```python
from build123d import *

# Parameters (mm, degrees)
SKETCH1_R                = 3.5
SKETCH1_R_2              = 1.5
SKETCH1_W                = 42
SKETCH1_H                = 22
BOSS_EXTRUDE1_DEPTH      = 10
CUT_EXTRUDE1_START       = 7
SKETCH2_R                = 3
CUT_EXTRUDE1_DEPTH       = 3
BOSS_EXTRUDE2_START      = -15
SKETCH4_R                = 5
BOSS_EXTRUDE2_DEPTH      = 10
BOSS_EXTRUDE3_DEPTH      = 15
BOSS_EXTRUDE3_DEPTH_BACK = 25
SKETCH4_3_R              = 5
SKETCH1_3_R              = 3.5
BOSS_EXTRUDE4_DEPTH      = 4
BOSS_EXTRUDE5_START      = -15
BOSS_EXTRUDE5_DEPTH      = 10
BOSS_EXTRUDE6_DEPTH      = 15
BOSS_EXTRUDE6_DEPTH_BACK = 25
SKETCH6_R                = 5
SKETCH6_R_2              = 3.5
BOSS_EXTRUDE7_START      = -19
SKETCH6_2_R              = 3.5
BOSS_EXTRUDE7_DEPTH      = 28


with BuildPart() as part:
    # Sketch1 → Boss-Extrude1 (new body)
    with BuildSketch(Plane.XY):
        Polygon((34, -15), (-29, -15), (-29, 15), (34, 15), (41.5, 15), (41.5, 7.5), (41.5, -7.5), (41.5, -15), align=None)
        with Locations((34, -7.5)):
            Circle(SKETCH1_R, mode=Mode.SUBTRACT)
        with Locations((34, 7.5)):
            Circle(SKETCH1_R, mode=Mode.SUBTRACT)
        with Locations((24.3, 5)):
            Circle(SKETCH1_R_2, mode=Mode.SUBTRACT)
        with Locations((24.3, -5)):
            Circle(SKETCH1_R_2, mode=Mode.SUBTRACT)
        with Locations(Location((-24.3, -5, 0), (0, 0, 180))):
            Circle(SKETCH1_R_2, mode=Mode.SUBTRACT)
        with Locations(Location((-24.3, 5, 0), (0, 0, 180))):
            Circle(SKETCH1_R_2, mode=Mode.SUBTRACT)
        Rectangle(SKETCH1_W, SKETCH1_H, mode=Mode.SUBTRACT)
    extrude(amount=BOSS_EXTRUDE1_DEPTH)

    # Sketch2 → Cut-Extrude1 (cut)
    with BuildSketch(Plane.XY.offset(CUT_EXTRUDE1_START)):
        with Locations((-24.3, 5)):
            Circle(SKETCH2_R)
        with Locations((-24.3, -5)):
            Circle(SKETCH2_R)
        with Locations((24.3, 5)):
            Circle(SKETCH2_R)
        with Locations((24.3, -5)):
            Circle(SKETCH2_R)
    extrude(amount=CUT_EXTRUDE1_DEPTH, mode=Mode.SUBTRACT)

    # Sketch4 → Boss-Extrude2 (add)
    # profile 1 of 3: a face of its own
    with BuildSketch(Plane(origin=(0, 0, 0), x_dir=(1, 0, 0), z_dir=(0, 1, 0)).offset(BOSS_EXTRUDE2_START)):
        with BuildLine():
            Line((41.5, 0), (41.5, 7))
            ThreePointArc((41.5, 7), (34.5, 14), (27.5, 7))
            Line((27.5, 7), (27.5, 0))
            Line((27.5, 0), (41.5, 0))
        make_face()
        with Locations((34.5, 7)):
            Circle(SKETCH4_R, mode=Mode.SUBTRACT)
    # profile 2 of 3: a face of its own
    with BuildSketch(Plane(origin=(0, 0, 0), x_dir=(1, 0, 0), z_dir=(0, 1, 0)).offset(BOSS_EXTRUDE2_START)):
        Polygon((-29, -10), (-29, 0), (27.5, 0), (41.5, 0), (41.5, -10), align=None)
    # profile 3 of 3: a face of its own
    with BuildSketch(Plane(origin=(0, 0, 0), x_dir=(1, 0, 0), z_dir=(0, 1, 0)).offset(BOSS_EXTRUDE2_START)):
        with BuildLine():
            Line((-29, 0), (-9.952221542, 0))
            ThreePointArc((-9.952221542, 0), (-7.49675311, 23.163932944), (6.211711403, 41.99675311))
            Line((6.211711403, 41.99675311), (3.068568225, 45.885281233))
            ThreePointArc((3.068568225, 45.885281233), (-16.210887038, 25.210644422), (-29, 0))
        make_face()
    extrude(amount=-BOSS_EXTRUDE2_DEPTH)

    # Sketch4<3> → Boss-Extrude3 (add, two sides: drawn at the far end of the back side and taken through both)
    with BuildSketch(Plane(origin=(0, 0, 0), x_dir=(1, 0, 0), z_dir=(0, 1, 0)).offset(-BOSS_EXTRUDE3_DEPTH_BACK)):
        with BuildLine():
            Line((41.5, 0), (41.5, 7))
            ThreePointArc((41.5, 7), (34.5, 14), (27.5, 7))
            Line((27.5, 7), (27.5, 0))
            Line((27.5, 0), (41.5, 0))
        make_face()
        with Locations((34.5, 7)):
            Circle(SKETCH4_3_R, mode=Mode.SUBTRACT)
    extrude(amount=BOSS_EXTRUDE3_DEPTH + BOSS_EXTRUDE3_DEPTH_BACK)

    # Sketch1<3> → Boss-Extrude4 (add)
    with BuildSketch(Plane.XY):
        with Locations((34, 7.5)):
            Circle(SKETCH1_3_R)
        with Locations((34, -7.5)):
            Circle(SKETCH1_3_R)
    extrude(amount=BOSS_EXTRUDE4_DEPTH)

    # Sketch5 → Boss-Extrude5 (add)
    with BuildSketch(Plane(origin=(0, 0, 0), x_dir=(1, 0, 0), z_dir=(0, 1, 0)).offset(BOSS_EXTRUDE5_START)):
        with BuildLine():
            Line((-7.556310354, 0), (-29, 0))
            ThreePointArc((-29, 0), (-16.210887038, 25.210644422), (3.068568225, 45.885281233))
            ThreePointArc((3.068568225, 45.885281233), (14.95066501, 52.529162568), (28.36797257, 54.831604973))
            Line((28.36797257, 54.831604973), (28.36797257, 51.580244948))
            Line((28.36797257, 51.580244948), (28.36797257, 49.056310354))
            ThreePointArc((28.36797257, 49.056310354), (27.851378801, 48.977742164), (27.335790025, 48.892828699))
            ThreePointArc((27.335790025, 48.892828699), (26.606861218, 46.521101207), (26.177213589, 44.077368115))
            ThreePointArc((26.177213589, 44.077368115), (25.629076173, 43.950056975), (25.082884112, 43.814642852))
            ThreePointArc((25.082884112, 43.814642852), (23.590633664, 45.796969038), (21.864411592, 47.579266955))
            ThreePointArc((21.864411592, 47.579266955), (21.366468722, 47.420852999), (20.870511092, 47.256329106))
            ThreePointArc((20.870511092, 47.256329106), (20.521576529, 44.799771926), (20.479502655, 42.318913548))
            ThreePointArc((20.479502655, 42.318913548), (19.95802957, 42.107422235), (19.439745475, 41.888232022))
            ThreePointArc((19.439745475, 41.888232022), (17.65576297, 43.612713083), (15.671980735, 45.103027328))
            ThreePointArc((15.671980735, 45.103027328), (15.204949771, 44.868668285), (14.740835409, 44.628585087))
            ThreePointArc((14.740835409, 44.628585087), (14.780487018, 42.147686811), (15.127022896, 39.690790112))
            ThreePointArc((15.127022896, 39.690790112), (14.645054541, 39.400326245), (14.167440286, 39.102757132))
            ThreePointArc((14.167440286, 39.102757132), (12.135653294, 40.526930621), (9.943158199, 41.688564712))
            ThreePointArc((9.943158199, 41.688564712), (9.518538992, 41.384031278), (9.097695935, 41.074300421))
            ThreePointArc((9.097695935, 41.074300421), (9.524957362, 38.630148998), (10.251570129, 36.257710929))
            ThreePointArc((10.251570129, 36.257710929), (9.820974163, 35.895426693), (9.395790198, 35.526805819))
            ThreePointArc((9.395790198, 35.526805819), (7.166228058, 36.615603857), (4.819006607, 37.419954507))
            ThreePointArc((4.819006607, 37.419954507), (4.447254693, 37.052745307), (4.080045493, 36.680993393))
            ThreePointArc((4.080045493, 36.680993393), (4.884396143, 34.333771942), (5.973194181, 32.104209802))
            ThreePointArc((5.973194181, 32.104209802), (5.604573307, 31.679025837), (5.242289071, 31.248429871))
            ThreePointArc((5.242289071, 31.248429871), (2.869851002, 31.975042638), (0.425699579, 32.402304065))
            ThreePointArc((0.425699579, 32.402304065), (0.115968722, 31.981461008), (-0.188564712, 31.556841801))
            ThreePointArc((-0.188564712, 31.556841801), (0.973069379, 29.364346706), (2.397242868, 27.332559714))
            ThreePointArc((2.397242868, 27.332559714), (2.099673755, 26.854945459), (1.809209888, 26.372977104))
            ThreePointArc((1.809209888, 26.372977104), (-0.647686811, 26.719512982), (-3.128585087, 26.759164591))
            ThreePointArc((-3.128585087, 26.759164591), (-3.368668285, 26.295050229), (-3.603027328, 25.828019265))
            ThreePointArc((-3.603027328, 25.828019265), (-2.112713083, 23.84423703), (-0.388232022, 22.060254525))
            ThreePointArc((-0.388232022, 22.060254525), (-0.607422235, 21.54197043), (-0.818913548, 21.020497345))
            ThreePointArc((-0.818913548, 21.020497345), (-3.299771926, 20.978423471), (-5.756329106, 20.629488908))
            ThreePointArc((-5.756329106, 20.629488908), (-5.920852999, 20.133531278), (-6.079266955, 19.635588408))
            ThreePointArc((-6.079266955, 19.635588408), (-4.296969038, 17.909366336), (-2.314642852, 16.417115888))
            ThreePointArc((-2.314642852, 16.417115888), (-2.450056975, 15.870923827), (-2.577368115, 15.322786411))
            ThreePointArc((-2.577368115, 15.322786411), (-5.021101207, 14.893138782), (-7.392828699, 14.164209975))
            ThreePointArc((-7.392828699, 14.164209975), (-7.477742164, 13.648621199), (-7.556310354, 13.13202743))
            ThreePointArc((-7.556310354, 13.13202743), (-5.525914856, 11.705870837), (-3.334554995, 10.542096605))
            ThreePointArc((-3.334554995, 10.542096605), (-3.382858682, 9.981445638), (-3.422854827, 9.420140853))
            ThreePointArc((-3.422854827, 9.420140853), (-5.769289812, 8.613498821), (-7.997787816, 7.522524415))
            ThreePointArc((-7.997787816, 7.522524415), (-8.001, 7), (-7.997787816, 6.477475585))
            ThreePointArc((-7.997787816, 6.477475585), (-5.769289812, 5.386501179), (-3.422854827, 4.579859147))
            ThreePointArc((-3.422854827, 4.579859147), (-3.382858682, 4.018554362), (-3.334554995, 3.457903395))
            ThreePointArc((-3.334554995, 3.457903395), (-5.525914856, 2.294129163), (-7.556310354, 0.86797257))
            Line((-7.556310354, 0.86797257), (-7.556310354, 0))
        make_face()
    extrude(amount=-BOSS_EXTRUDE5_DEPTH)

    # Sketch6 → Boss-Extrude6 (add, two sides: drawn at the far end of the back side and taken through both)
    with BuildSketch(Plane(origin=(0, 0, 0), x_dir=(1, 0, 0), z_dir=(0, 1, 0)).offset(-BOSS_EXTRUDE6_DEPTH_BACK)):
        with Locations((34.5, 7)):
            Circle(SKETCH6_R)
        with Locations(Location((34.5, 7, 0), (0, 0, 90))):
            Circle(SKETCH6_R_2, mode=Mode.SUBTRACT)
    extrude(amount=BOSS_EXTRUDE6_DEPTH + BOSS_EXTRUDE6_DEPTH_BACK)

    # Sketch6<2> → Boss-Extrude7 (add)
    with BuildSketch(Plane(origin=(0, 0, 0), x_dir=(1, 0, 0), z_dir=(0, 1, 0)).offset(BOSS_EXTRUDE7_START)):
        with Locations(Location((34.5, 7, 0), (0, 0, 90))):
            Circle(SKETCH6_2_R)
    extrude(amount=BOSS_EXTRUDE7_DEPTH)


solid = part.part
```
For this review, take the finished solid that the model builds, in its own axes (mm). A direction names the side the tool comes from. Coordinates: 2 decimals unless noted, no trailing zeros. Write each loop counter-clockwise with the first axis right and the second up, starting at its lowest first coordinate (ties: lowest second). Pieces come first, ordered by that corner, then holes. Notation, with made-up numbers: (-8.5, -0.75) -> (37.5, -0.75) arc R24 cw to (37.5, 9.25) -> close; hole circle Ø2 at (-24, 52.25). An arc over 180 degrees is marked (long way). Put each result on its own line as item: value.
Q1. Tool access review of faces 4 (the cylindrical face through (-5.556, -19.93, -11.724)), 5 (the cylindrical face through (-24.691, -2.026, 8.479)), 6 (the cylindrical face through (-2.135, -19.93, -23.871)): name each direction out of +Z, -Z, +X, -X, +Y, -Y from which nothing blocks a thin tool from reaching the whole face with its end or side.
From the geometry:
face 4: +Y, -Y
face 5: +Z
face 6: +X, +Y, -Y
Q2. Take a section at D-D, the plane x = 36.5. State the section outline as (y, z) points, then the cut area to 3 significant figures.
From the geometry:
outline: (-25, -13.71) -> (15, -13.71) -> (15, -9.87) -> (9, -9.87) -> (9, -4.13) -> (15, -4.13) -> (15, 10) -> (9.95, 10) -> (9.95, 4) -> (5.05, 4) -> (5.05, 10) -> (-5.05, 10) -> (-5.05, 4) -> (-9.95, 4) -> (-9.95, 10) -> (-25, 10) -> (-25, -4.13) -> (-19, -4.13) -> (-19, -9.87) -> (-25, -9.87) -> close
area: 821 mm2
Q3. Take a section at A-A, the plane y = -1. State the section outline as (x, z) points, then the cut area to 3 significant figures.
From the geometry:
outline: (-29, 0) -> (-21, 0) -> (-21, 10) -> (-29, 10) -> close; (21, 0) -> (27.5, 0) -> (27.5, -7) arc R7 ccw to (41.5, -7) -> (41.5, 10) -> (21, 10) -> close
area: 460 mm2
Q4. Wall thickness on L1, parallel to Y at x = 34, z = 7; L2, parallel to Y at x = -24.3, z = 8.15; L3, parallel to Z at x = 34.5, y = 10.6: over which ranges is each line inside the solid? List them lowest first.
From the geometry:
L1: y = -25 to -11, -4 to 4, 11 to 15
L2: y = -25 to -8, -2 to 2, 8 to 15
L3: z = -14 to -10.5, -3.5 to 4
Q5. Clearance check with flat-ended pins moving along their axes: pin 1 Ø8 at (x, y) = (24.3, -5) entering from -Z; pin 2 Ø3.5 at (x, y) = (-24.3, 5) entering from -Z; pin 3 Ø3.5 at (x, z) = (35.5, -7) entering from +Y. State where each tip first meets the part, or that it passes through.
From the geometry:
pin 1: stops at z = -10.25
pin 2: stops at z = 0
pin 3: stops at y = 9
Q6. Take a section at B-B, the plane x = -24.3. State the section outline as (y, z) points, then the cut area to 3 significant figures.
From the geometry:
outline: (-25, -11.43) -> (-15, -11.43) -> (-15, 0) -> (-6.5, 0) -> (-6.5, 7) -> (-8, 7) -> (-8, 10) -> (-25, 10) -> close; (-3.5, 0) -> (3.5, 0) -> (3.5, 7) -> (2, 7) -> (2, 10) -> (-2, 10) -> (-2, 7) -> (-3.5, 7) -> close; (6.5, 0) -> (15, 0) -> (15, 10) -> (8, 10) -> (8, 7) -> (6.5, 7) -> close
area: 436 mm2
Q7. The part is to be moulded in two halves that separate along Z. For faces 1 (the flat face through (15, -14, 10)), 2 (the flat face through (21, 0, 5)), 3 (the cylindrical face through (17.68, -19.93, -43.59)), say which applies: +Z half, -Z half, draft (parallel to the pull), parting line (faces both ways), or undercut.
From the geometry:
face 1: +Z half
face 2: draft
face 3: undercut
Q8. Take a section at C-C, the plane y = 5. Count the separate pieces of the cut face and the enclosed holes in it, then the cut area to 3 significant figures.
From the geometry:
separate pieces: 4
enclosed holes: 0
area: 353 mm2
